```python
from build123d import *

# Parameters (mm, degrees)
SKETCH004_W     = 200
SKETCH004_H     = 200
PAD001_DEPTH    = 150
SKETCH005_W     = 195
SKETCH005_H     = 195
POCKET002_DEPTH = 147.5
FILLET_R        = 6
FILLET001_R     = 3.5


with BuildPart() as part:
    # Sketch004 → Pad001 (new body)
    with BuildSketch(Plane.XY):
        Rectangle(SKETCH004_W, SKETCH004_H)
    extrude(amount=PAD001_DEPTH)

    # Sketch005 (on Face6 of Pad001) → Pocket002 (cut)
    with BuildSketch(Plane.XY.offset(150)):
        Rectangle(SKETCH005_W, SKETCH005_H)
    extrude(amount=-POCKET002_DEPTH, mode=Mode.SUBTRACT)

    # Fillet
    fillet_edges = [part.edges().sort_by_distance(p)[0] for p in [
        (-100, -100, 75),
        (100, -100, 75),
        (100, 100, 75),
        (-100, 100, 75),
    ]]
    fillet(fillet_edges, radius=FILLET_R)

    # Fillet001
    fillet001_edges = [part.edges().sort_by_distance(p)[0] for p in [
        (97.5, 97.5, 76.25),
        (-97.5, 97.5, 76.25),
        (97.5, -97.5, 76.25),
        (-97.5, -97.5, 76.25),
    ]]
    fillet(fillet001_edges, radius=FILLET001_R)


solid = part.part
```
CAD build for the part. Positions are in the model's coordinates, mm. A direction names the side the tool comes from. Coordinates: 2 decimals unless noted, no trailing zeros. Order: outer loops, then holes, each group sorted by start corner. A loop starts at its lowest first (then second) coordinate and runs counter-clockwise, first axis right, second up.
(1) Drill centre lines: L1, parallel to Y at x = -9, z = 125; L2, parallel to Z at x = -85, y = -2. Where is each one in solid material? Low to high.
Solution:
L1: y = -100 to -97.5, 97.5 to 100
L2: z = 0 to 2.5
(2) Pin check, flat tip, straight feed: pin 1 Ø5 at (x, y) = (8, -45) entering from +Z. Stop position of the tip, or through.
Solution:
pin 1: stops at z = 2.5
(3) Mould opens along X. For faces 3 (the face through (-1, -97.5, 77)), 4 (the face through (-100, -1, 74)), 5 (the face through (-1, 1, 0)) say: released by +X, released by -X, zero draft, split by the parting line, or undercut.
Solution:
face 3: undercut
face 4: released by -X
face 5: zero draft
(4) Saw through at B-B, the plane z = 106. Write the cut outline in (x, y).
Solution:
outline: (-100, -94) arc R6 ccw to (-94, -100) - (94, -100) arc R6 ccw to (100, -94) - (100, 94) arc R6 ccw to (94, 100) - (-94, 100) arc R6 ccw to (-100, 94) - close; hole (-97.5, -94) arc R3.5 ccw to (-94, -97.5) - (94, -97.5) arc R3.5 ccw to (97.5, -94) - (97.5, 94) arc R3.5 ccw to (94, 97.5) - (-94, 97.5) arc R3.5 ccw to (-97.5, 94) - close
(5) Which spindle directions (+Z, -Z, +X, -X, +Y, -Y) get a long thin tool onto all of the face, cutting with end or side? Do faces 1 (the face through (97.5, -1, 77)), 2 (the face through (-98.289, -98.196, 76.05)). Say none if no direction does.
Solution:
face 1: +Z
face 2: +Z, -Z, -X, -Y
(6) Saw through at A-A, the plane x = -85.5. Write the cut outline in (y, z).
Solution:
outline: (-100, 0) - (100, 0) - (100, 150) - (97.5, 150) - (97.5, 2.5) - (-97.5, 2.5) - (-97.5, 150) - (-100, 150) - close
